Part model, mm, in its own coordinate system. A direction names the side the tool comes from. Give positions to 0.01 mm unless a question says otherwise; leave off trailing zeros. Write each loop counter-clockwise with the first axis right and the second up, starting at its lowest first coordinate (ties: lowest second). Pieces come first, ordered by that corner, then holes. Notation, with made-up numbers: (68, 87.5) - (123, 87.5) arc R19 ccw to (123, 98.5) - close; hole circle Ø10 at (67, 34.25). An arc over 180 degrees is marked (long way). Answer as a JSON object with one key per item and string values. Group by question number.
```python
from build123d import *

# Parameters (mm, degrees)
CROQUIS1_W              = 75
CROQUIS1_H              = 75
CROQUIS1_R              = 5
SALIENTE_EXTRUIR1_DEPTH = 9.525
CROQUIS2_R              = 10
CORTAR_EXTRUIR1_DEPTH   = 5


with BuildPart() as part:
    # Croquis1 → Saliente-Extruir1 (new body)
    with BuildSketch(Plane(origin=(0, 0, 0), x_dir=(1, 0, 0), z_dir=(0, 1, 0))):
        Rectangle(CROQUIS1_W, CROQUIS1_H)
        with Locations(Location((0, 9.022258823, 0), (0, 0, 90))):
            Circle(CROQUIS1_R, mode=Mode.SUBTRACT)
    extrude(amount=SALIENTE_EXTRUIR1_DEPTH)

    # Croquis2 → Cortar-Extruir1 (cut)
    with BuildSketch(Plane(origin=(0, 9.525, 0), x_dir=(1, 0, 0), z_dir=(0, 1, 0))):
        with Locations(Location((0, 9.022258823, 0), (0, 0, 270))):
            Circle(CROQUIS2_R)
    extrude(amount=-CORTAR_EXTRUIR1_DEPTH, mode=Mode.SUBTRACT)


solid = part.part
```
1) Saw through at B-B (y = 6). List the corners of the cut face in (x, z).
2) Drop flat-ended pins along their axis: P1, Ø12, axis at x = 0, z = -9.02, coming from the +Y side (3 decimals); P2, Ø9, axis at x = 0, z = -9.02, coming from the -Y side. Give the stop position or say it passes through.
3) Which spindle directions (+Z, -Z, +X, -X, +Y, -Y) get a long thin tool onto all of the face, cutting with end or side? Do faces 1 (the flat face through (-1, 5, 37.5)), 2 (the cylindrical face through (-9.762, 7.06, -11.19)). Say none if no direction does.
4) Two-plate mould, pull along X, no slides. Class faces 3 (the flat face through (-1, 5, -37.5)), 4 (the flat face through (5, 4.525, -7)), 5 (the flat face through (-37.5, 5, 1)): +X half, -X half, draft (parallel to the pull), parting line (faces both ways), or undercut.
5) Drill centre line: line 1 along X through (y, z) = (2.5, -10). Where is it in solid material? Low to high. Write a range as from..to.
6) Saw through at A-A (x = 0). List the corners of the cut face in (y, z) (3 decimals).
7) Saw through at C-C (z = -3). List the corners of the cut face in (x, y) (3 decimals), and give its area (3 significant figures).
Checks:
{
 "1": {"outline": "(-37.5, -37.5) - (37.5, -37.5) - (37.5, 37.5) - (-37.5, 37.5) - close; hole circle Ø20 at (0, -9.02)"},
 "2": {"P1": "y = 4.525", "P2": "through"},
 "3": {"face 1": "+Z, +X, -X, +Y, -Y", "face 2": "+Y"},
 "4": {"face 3": "draft", "face 4": "undercut", "face 5": "-X half"},
 "5": {"line 1": "-37.5..-4.9, 4.9..37.5"},
 "6": {"outline": "(0, -37.5) - (9.525, -37.5) - (9.525, -19.022) - (4.525, -19.022) - (4.525, -14.022) - (0, -14.022) - close; (0, -4.022) - (4.525, -4.022) - (4.525, 0.978) - (9.525, 0.978) - (9.525, 37.5) - (0, 37.5) - close"},
 "7": {"outline": "(-37.5, 0) - (37.5, 0) - (37.5, 9.525) - (7.983, 9.525) - (7.983, 4.525) - (-7.983, 4.525) - (-7.983, 9.525) - (-37.5, 9.525) - close", "area": "635 mm2"}
}
